```python
from build123d import *

# Parameters (mm, degrees)
SALIENTE_EXTRUIR1_DEPTH = 10
CROQUIS2_R              = 100
CORTAR_EXTRUIR1_DEPTH   = 10


with BuildPart() as part:
    # Croquis1 → Saliente-Extruir1 (new body)
    with BuildSketch(Plane.XY):
        with BuildLine():
            ThreePointArc((-72.516892967, 473.757277013), (0, 490), (72.516892967, 473.757277013))
            ThreePointArc((72.516892967, 473.757277013), (106.066017178, 426.066017178), (153.757277013, 392.516892967))
            ThreePointArc((153.757277013, 392.516892967), (170, 320), (153.757277013, 247.483107033))
            ThreePointArc((153.757277013, 247.483107033), (106.066017178, 213.933982822), (72.516892967, 166.242722987))
            ThreePointArc((72.516892967, 166.242722987), (0, 150), (-72.516892967, 166.242722987))
            ThreePointArc((-72.516892967, 166.242722987), (-106.066017178, 213.933982822), (-153.757277013, 247.483107033))
            ThreePointArc((-153.757277013, 247.483107033), (-170, 320), (-153.757277013, 392.516892967))
            ThreePointArc((-153.757277013, 392.516892967), (-106.066017178, 426.066017178), (-72.516892967, 473.757277013))
        make_face()
    extrude(amount=SALIENTE_EXTRUIR1_DEPTH)

    # Croquis2 → Cortar-Extruir1 (cut)
    with BuildSketch(Plane.XY.offset(10)):
        with Locations((0, 320)):
            Circle(CROQUIS2_R)
    extrude(amount=-CORTAR_EXTRUIR1_DEPTH, mode=Mode.SUBTRACT)


solid = part.part
```
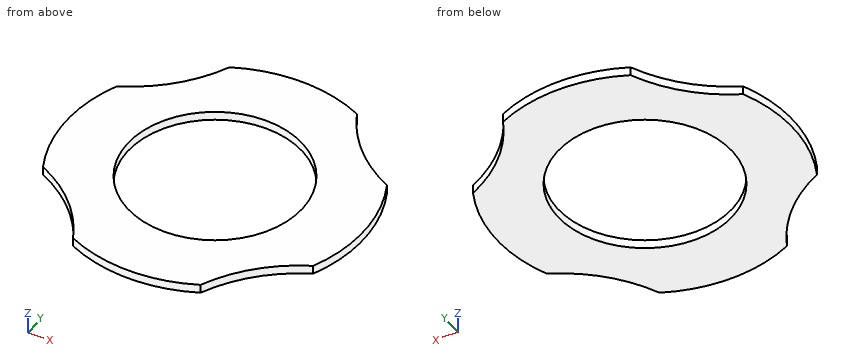
Here's how the part is built. I have some questions about the finished solid (model axes, mm). Coordinates: 2 decimals unless noted, no trailing zeros. Order: outer loops, then holes, each group sorted by start corner. A loop starts at its lowest first (then second) coordinate and runs counter-clockwise, first axis right, second up.
1) Imagine slicing it at C-C on z = 6.5. List the corners of the cut face in (x, y) for me.
2) Imagine slicing it at D-D on x = -119. List the corners of the cut face in (y, z) for me.
3) Will these pins go through, and if not, where does the flat tip stop? pin 1 (2 mm diameter, centred on x = 29.5, z = 5, fed in from -Y); pin 2 (4 mm diameter, centred on x = 92, z = 3, fed in from +Y); pin 3 (6 mm diameter, centred on x = -57, z = 7.5, fed in from -Y).
4) Imagine slicing it at B-B on y = 320. List the corners of the cut face in (x, z) for me.
5) Imagine slicing it at A-A on x = 0. List the corners of the cut face in (y, z) for me, and give its area (3 significant figures).
6) I need wall thicknesses on line 1 (X direction, y = 322, z = 4); line 2 (X direction, y = 280, z = 3.25); line 3 (Y direction, x = 22.5, z = 4.25). Which ranges of each line are inside material? Lowest first, please.
Response values:
1. outline: (-153.76, 247.48) arc R170 cw to (-72.52, 166.24) arc R170 ccw to (72.52, 166.24) arc R170 cw to (153.76, 247.48) arc R170 ccw to (153.76, 392.52) arc R170 cw to (72.52, 473.76) arc R170 ccw to (-72.52, 473.76) arc R170 cw to (-153.76, 392.52) arc R170 ccw to start; hole circle Ø200 at (0, 320)
2. outline: (225.61, 0) - (414.39, 0) - (414.39, 10) - (225.61, 10) - close
3. pin 1: stops at y = 152.41
3. pin 2: stops at y = 444.64
3. pin 3: stops at y = 158.8
4. outline: (-170, 0) - (-100, 0) - (-100, 10) - (-170, 10) - close; (100, 0) - (170, 0) - (170, 10) - (100, 10) - close
5. outline: (150, 0) - (220, 0) - (220, 10) - (150, 10) - close; (420, 0) - (490, 0) - (490, 10) - (420, 10) - close
5. area: 1,400 mm2
6. line 1: x = -169.99 to -99.98, 99.98 to 169.99
6. line 2: x = -165.23 to -91.65, 91.65 to 165.23
6. line 3: y = 151.5 to 222.56, 417.44 to 488.5
